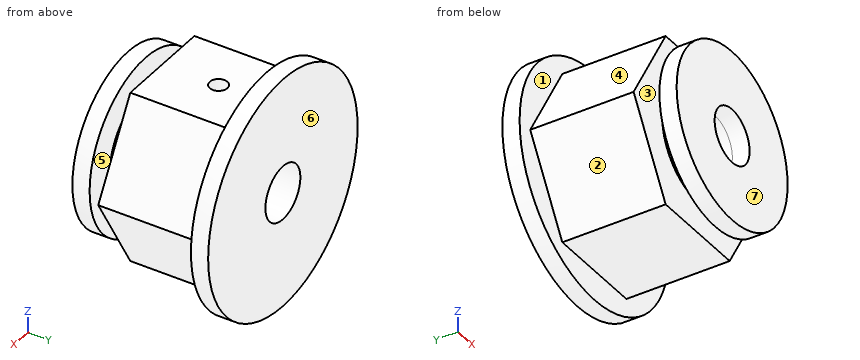
Autodesk Inventor part; units mm, degrees
ref_plane "YZ Plane" through (0, 0, 0) normal (1, 0, 0) x (0, 1, 0)
ref_plane "XZ Plane" through (0, 0, 0) normal (0, 1, 0) x (-1, 0, 0)
ref_plane "XY Plane" through (0, 0, 0) normal (0, 0, 1) x (1, 0, 0)
sketch "Esquisse1" plane through (0, 0, 0) normal (0, 1, 0) x (-1, 0, 0)
  circle A0 centre (0, 0) radius 2
  line L0 (7.3323, 0) -> (3.6662, -6.35)
  line L1 (3.6662, -6.35) -> (-3.6662, -6.35)
  line L2 (-3.6662, -6.35) -> (-7.3323, 0)
  line L3 (-7.3323, 0) -> (-3.6662, 6.35)
  line L4 (-3.6662, 6.35) -> (3.6662, 6.35)
  line L5 (3.6662, 6.35) -> (7.3323, 0)
  dimension "d0" = 12.7
  dimension "d1" = 4
extrude "Extrusion1" add sketch "Esquisse1" along normal blind 7.62
sketch "Esquisse2" plane through (0, 7.62, 0) normal (0, 1, 0) x (1, 0, 0)
  circle A0 centre (0, 0) radius 8.5509
  circle A1 centre (0, 0) radius 2
extrude "Extrusion2" add sketch "Esquisse2" along normal blind 1.27
sketch "Esquisse3" plane through (0, 0, 0) normal (0, -1, 0) x (1, 0, 0)
  circle A0 centre (0, 0) radius 4.0595
  circle A1 centre (0, 0) radius 2
extrude "Extrusion3" add sketch "Esquisse3" along normal blind 1.27
sketch "Esquisse4" plane through (0, -1.27, 0) normal (0, -1, 0) x (1, 0, 0)
  circle A0 centre (0, 0) radius 6.35
  line L0 (7.3323, 0) -> (3.6662, 6.35)
  circle A1 centre (0, 0) radius 2
extrude "Extrusion4" add sketch "Esquisse4" along normal blind 1.27
sketch "Esquisse5" plane through (-3.6662, 0, 6.35) normal (0, 0, 1) x (1, 0, 0)
  circle A0 centre (3.6662, 4.1459) radius 0.6492
  point P0 (3.6662, 0)
extrude "Extrusion5" cut sketch "Esquisse5" against normal blind 6
properties part number "T40_hub_40mm_1screw"
Can you work these out from the model? Positions are in its coordinate system, mm. Face numbers are marked on the shaded views. A direction names the side the tool comes from. Coordinates: 2 decimals unless noted, no trailing zeros. Loops run counter-clockwise (first coordinate to the right, second up) from the corner with the lowest first, then second, coordinate; pieces in that order, holes last.
1) Imagine slicing it at B-B on z = -1. List the corners of the cut face in (x, y) for me, plus the area to 3 significant figures.
2) Thinking about a two-plate mould opening in Y: for the marked faces 4, 5, 6 and 7, which applies, pulls with the +Y half, pulls with the -Y half, needs draft (parallel to the pull), parting line crosses it, or undercut?
3) I need wall thicknesses on probe 1 along Y at (x, z) = (-4, -1.75); probe 2 along Y at (x, z) = (0, 3.45); probe 3 along Y at (x, z) = (7, -3.25). Which ranges of each line are inside material? Lowest first, please.
4) Imagine slicing it at D-D on z = 3. List the corners of the cut face in (x, y) for me.
5) Which directions (+Z, -Z, +X, -X, +Y, -Y) give clear straight access to the entire face, cutting with the end or side of a thin tool? Please do the marked faces 1, 2 and 3.
6) Imagine slicing it at C-C on y = 2. List the corners of the cut face in (x, z) for me.
7) For pin 1 (3.5 mm diameter, centred on x = -1.5, y = 4, fed in from +Z); pin 2 (2 mm diameter, centred on x = 2, y = 0, fed in from -Z); pin 3 (3 mm diameter, centred on y = 3, z = -6.5, fed in from -X), each with a flat end and sliding along its axis, tell me the tip position at first contact or that it passes through.
Completed:
1. outline: (-8.49, 7.62) - (-6.75, 7.62) - (-6.75, 0) - (-3.93, 0) - (-3.93, -1.27) - (-6.27, -1.27) - (-6.27, -2.54) - (-1.73, -2.54) - (-1.73, 8.89) - (-8.49, 8.89) - close; (1.73, -2.54) - (6.27, -2.54) - (6.27, -1.27) - (3.93, -1.27) - (3.93, 0) - (6.75, 0) - (6.75, 7.62) - (8.49, 7.62) - (8.49, 8.89) - (1.73, 8.89) - close
1. area: 111 mm2
2. face 4: needs draft
2. face 5: undercut
2. face 6: pulls with the +Y half
2. face 7: pulls with the -Y half
3. probe 1: y = -2.54 to -1.27, 0 to 8.89
3. probe 2: y = -2.54 to 3.5, 4.8 to 8.89
3. probe 3: y = 7.62 to 8.89
4. outline: (-8.01, 7.62) - (-5.6, 7.62) - (-5.6, 0) - (-2.73, 0) - (-2.73, -1.27) - (-5.6, -1.27) - (-5.6, -2.54) - (5.6, -2.54) - (5.6, -1.27) - (2.73, -1.27) - (2.73, 0) - (5.6, 0) - (5.6, 7.62) - (8.01, 7.62) - (8.01, 8.89) - (-8.01, 8.89) - close; hole circle Ø1.3 at (0, 4.15)
5. face 1: -Y
5. face 2: -Z, -X, -Y
5. face 3: none
6. outline: (-7.33, 0) - (-3.67, -6.35) - (3.67, -6.35) - (7.33, 0) - (3.67, 6.35) - (-3.67, 6.35) - close; hole circle Ø4 at (0, 0)
7. pin 1: stops at z = 6.35
7. pin 2: stops at z = -6.35
7. pin 3: stops at x = -4.45
